Could you check a few things on this drawing? It's one solid part, dimensions in mm from its lowest x, y, z. Give positions to 0.01 mm unless a question says otherwise; leave off trailing zeros. Loops run counter-clockwise (first coordinate to the right, second up) from the corner with the lowest first, then second, coordinate; pieces in that order, holes last. Notation, with made-up numbers: M 75,33.5 L 111,33.5 A17 cw 111,57.5 Z; hole C 13,65 d9. An arc over 180 degrees is marked long. Answer in a Markdown table with one row per item. Add a question column.
1. Thinking about a two-plate mould opening in X: for the marked faces 1, 2 and 3, which applies, released by +X, released by -X, zero draft, split by the parting line, or undercut?
2. If we section it at C-C on z = 7: List the corners of the cut face in (x, y) for me, then the cut area to 3 significant figures.
3. If we section it at B-B on y = 18: List the corners of the cut face in (x, z) for me.
4. I need wall thicknesses on line 1 along Y through (x, z) = (73, 3.55); line 2 along Z through (x, y) = (79, 7); line 3 along X through (y, z) = (94.5, 2). Which ranges of each line are inside material? Lowest first, please. Write a range as from..to.
5. If we section it at A-A on x = 93.5: List the corners of the cut face in (y, z) for me.
6. I'm going to push flat-ended pins straight in: pin 1 Ø5 at (x, y) = (105.5, 96.5) entering from +Z; pin 2 Ø2 at (y, z) = (33, 11.5) entering from +X; pin 3 Ø5 at (y, z) = (61.5, 3) entering from +X. Where does each tip first touch, or does it pass through?
7. If we section it at D-D on x = 29.5: List the corners of the cut face in (y, z) for me.
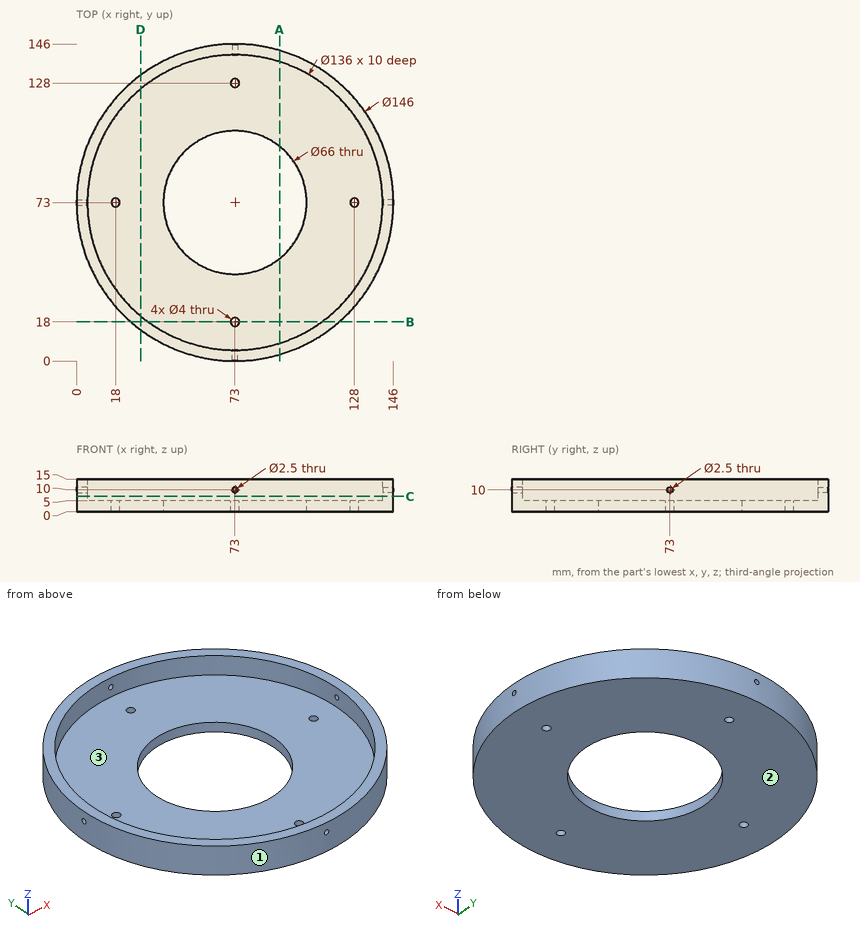
Results:
| question | item | result |
|---|---|---|
| 1 | face 1 | split by the parting line |
| 1 | face 2 | zero draft |
| 1 | face 3 | undercut |
| 2 | outline | C 73,73 d146; hole C 73,73 d136 |
| 2 | area | 2,210 mm2 |
| 3 | outline | M 25,0 L 71,0 L 71,5 L 33.01,5 L 33.01,15 L 25,15 Z; M 75,0 L 121,0 L 121,15 L 112.99,15 L 112.99,5 L 75,5 Z |
| 4 | line 1 | 0..16, 20..40, 106..126, 130..146 |
| 4 | line 2 | 0..5 |
| 4 | line 3 | 3.24..47.97, 98.03..142.76 |
| 5 | outline | M 2.94,0 L 47.14,0 L 47.14,5 L 8.16,5 L 8.16,15 L 2.94,15 Z; M 98.86,0 L 143.06,0 L 143.06,15 L 137.84,15 L 137.84,5 L 98.86,5 Z |
| 6 | pin 1 | z = 5 |
| 6 | pin 2 | x = 134.71 |
| 6 | pin 3 | x = 145.44 |
| 7 | outline | M 14.38,0 L 131.62,0 L 131.62,15 L 125.27,15 L 125.27,5 L 20.73,5 L 20.73,15 L 14.38,15 Z |
